Answer from the drawing. Dimensions are ordinates in mm from the lowest x, y and z of the part. A direction names the side the tool comes from. Give positions to 0.01 mm unless a question says otherwise; leave off trailing zeros. Order: outer loops, then holes, each group sorted by start corner. A loop starts at its lowest first (then second) coordinate and runs counter-clockwise, first axis right, second up. Notation, with made-up numbers: (22, -31) - (71, -31) arc R11 cw to (71, -14) - close; hole circle Ø10 at (33.25, 15.5). An arc over 180 degrees is marked (long way). Answer in a Markdown table with one row per item.
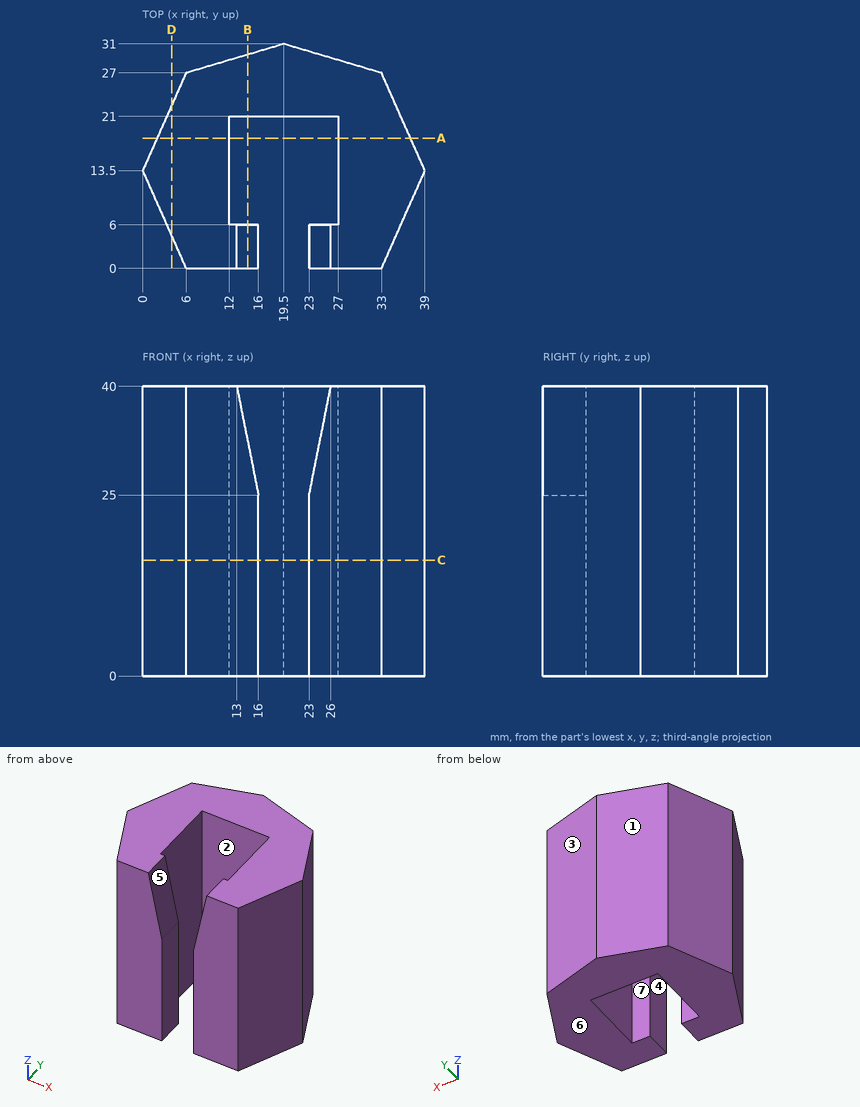
Item 1: Find section B-B on x = 14.5. Write down the section's boundary in (y, z).
Answer block:
| item | result |
|---|---|
| outline | (0, 0) - (6, 0) - (6, 32.5) - (0, 32.5) - close; (21, 0) - (29.52, 0) - (29.52, 40) - (21, 40) - close |
Item 2: Find section C-C on z = 16. Write down the section's boundary in (x, y), then the cut area to 3 significant figures.
Answer block:
| item | result |
|---|---|
| outline | (0, 13.5) - (6, 0) - (16, 0) - (16, 6) - (12, 6) - (12, 21) - (27, 21) - (27, 6) - (23, 6) - (23, 0) - (33, 0) - (39, 13.5) - (33, 27) - (19.5, 31) - (6, 27) - close |
| area | 678 mm² |
Item 3: Find section A-A on y = 18. Write down the section's boundary in (x, z), then the cut area to 3 significant figures.
Answer block:
| item | result |
|---|---|
| outline | (2, 0) - (12, 0) - (12, 40) - (2, 40) - close; (27, 0) - (37, 0) - (37, 40) - (27, 40) - close |
| area | 800 mm² |
Item 4: Which of the six approach directions +Z, -Z, +X, -X, +Y, -Y give full straight-line access (tool end or side, diameter ignored) to the marked faces 4, 5, 6 and 7?
Answer block:
| item | result |
|---|---|
| face 4 | +Z, -Z, -Y |
| face 5 | +Z, -Y |
| face 6 | -Z, +X, -X, +Y, -Y |
| face 7 | +Z, -Z |
Item 5: Each of these flat-tipped pins is pushed along its axis until it touches: P1, Ø2, axis at x = 25.5, z = 17.5, coming from the +Y side; P2, Ø7.5, axis at y = 10.5, z = 19.5, coming from the -X side; P3, Ø4, axis at x = 25, z = 20.5, coming from the +Y side; P4, Ø3, axis at x = 25, z = 36, coming from the +Y side. Where does it stop, or does it pass through?
Answer block:
| item | result |
|---|---|
| P1 | y = 29.52 |
| P2 | x = 0 |
| P3 | y = 29.96 |
| P4 | y = 29.81 |
Item 6: Find section D-D on x = 4. Write down the section's boundary in (y, z), then the cut area to 3 significant figures.
Answer block:
| item | result |
|---|---|
| outline | (4.5, 0) - (22.5, 0) - (22.5, 40) - (4.5, 40) - close |
| area | 720 mm² |
Item 7: Consider line 1 (X direction, y = 8, z = 8.5); line 2 (X direction, y = 20, z = 35.5); line 3 (Y direction, x = 20, z = 33). Determine where each line is inside the solid, lowest interval first.
Answer block:
| item | result |
|---|---|
| line 1 | 2.44 to 12, 27 to 36.56 |
| line 2 | 2.89 to 12, 27 to 36.11 |
| line 3 | 21 to 30.85 |
Item 8: Determine the mould class of the marked faces 1, 2 and 3 for opening direction X: pulls with the +X half, pulls with the -X half, needs draft (parallel to the pull), parting line crosses it, or undercut.
Answer block:
| item | result |
|---|---|
| face 1 | pulls with the -X half |
| face 2 | undercut |
| face 3 | pulls with the +X half |
